The model under review builds one solid part; all positions refer to its coordinate system, in mm. Round coordinates to 2 decimals unless told otherwise and drop trailing zeros. Write each loop counter-clockwise with the first axis right and the second up, starting at its lowest first coordinate (ties: lowest second). Pieces come first, ordered by that corner, then holes. Notation, with made-up numbers: (58.25, 83) -> (77.25, 83) arc R38 ccw to (77.25, 121) -> close; hole circle Ø7 at (85, -28.5). An arc over 180 degrees is marked (long way). Return JSON: item names as keys, results as strings. Group by question number.
1. For line 1 along X through (y, z) = (-8.25, 0); line 2 along Z through (x, y) = (-29.5, -6.5); line 3 along Z through (x, y) = (-42.5, -7.75), list the stretches that pass through material, from the lowest coordinate up. Write a range as from..to.
2. Take a section at A-A, the plane x = 0. Write out the cut boundary in (y, z), then the cut area to 3 significant figures.
3. Mouldability with a two-part tool opening along X and no side actions: class faces 1 (the cylindrical face through (43.339, -6.261, -43.477)), 2 (the cylindrical face through (-35.265, -6.261, -0.688)), 3 (the flat face through (-1, -6, -50.8)), 4 (the flat face through (-50.8, -6, 1)) as pulls with the +X half, pulls with the -X half, needs draft (parallel to the pull), parting line crosses it, or undercut.
4. Take a section at B-B, the plane z = 0. Write out the cut boundary in (x, y).
from build123d import *

# Parameters (mm, degrees)
SKETCH1_W           = 101.6
SKETCH1_H           = 101.6
BOSS_EXTRUDE1_DEPTH = 12.7
SKETCH3_R           = 3.175
SKETCH3_R_2         = 2.2479
SKETCH3_R_3         = 1.7272
CUT_EXTRUDE1_DEPTH  = 73.955945611


with BuildPart() as part:
    # Sketch1 → Boss-Extrude1 (new body)
    with BuildSketch(Plane(origin=(0, 0, 0), x_dir=(1, 0, 0), z_dir=(0, 1, 0))):
        Rectangle(SKETCH1_W, SKETCH1_H)
    extrude(amount=-BOSS_EXTRUDE1_DEPTH)

    # Sketch3 → Cut-Extrude1 (cut, through all)
    with BuildSketch(Plane(origin=(0, 0, 0), x_dir=(1, 0, 0), z_dir=(0, 1, 0))):
        with Locations(Location((17.8435508, 0, 0), (0, 0, 270))):
            Circle(SKETCH3_R)
        with Locations(Location((-32.16507791, 0, 0), (0, 0, 270))):
            Circle(SKETCH3_R)
        with Locations(Location((-41.819743879, 41.819743879, 0), (0, 0, 270))):
            Circle(SKETCH3_R_2)
        with Locations(Location((41.819743879, 41.819743879, 0), (0, 0, 270))):
            Circle(SKETCH3_R_2)
        with Locations(Location((41.819743879, -41.819743879, 0), (0, 0, 270))):
            Circle(SKETCH3_R_2)
        with Locations(Location((-41.819743879, -41.819743879, 0), (0, 0, 270))):
            Circle(SKETCH3_R_2)
        with Locations(Location((0, 0, 0), (0, 0, 270))):
            Circle(SKETCH3_R_3)
    extrude(amount=-CUT_EXTRUDE1_DEPTH, mode=Mode.SUBTRACT)


solid = part.part
Output:
{
 "1": {"line 1": "x = -50.8..-35.34, -28.99..-1.73, 1.73..14.67, 21.02..50.8", "line 2": "z = -50.8..-1.73, 1.73..50.8", "line 3": "z = -50.8..-43.96, -39.68..39.68, 43.96..50.8"},
 "2": {"outline": "(-12.7, -50.8) -> (0, -50.8) -> (0, -1.73) -> (-12.7, -1.73) -> close; (-12.7, 1.73) -> (0, 1.73) -> (0, 50.8) -> (-12.7, 50.8) -> close", "area": "1,250 mm^2"},
 "3": {"face 1": "undercut", "face 2": "undercut", "face 3": "needs draft", "face 4": "pulls with the -X half"},
 "4": {"outline": "(-50.8, -12.7) -> (-35.34, -12.7) -> (-35.34, 0) -> (-50.8, 0) -> close; (-28.99, -12.7) -> (-1.73, -12.7) -> (-1.73, 0) -> (-28.99, 0) -> close; (1.73, -12.7) -> (14.67, -12.7) -> (14.67, 0) -> (1.73, 0) -> close; (21.02, -12.7) -> (50.8, -12.7) -> (50.8, 0) -> (21.02, 0) -> close"}
}
